from build123d import *

# Parameters (mm, degrees)
F0_W         = 35
F0_H         = 12
F0_W_2       = 12
F0_H_2       = 2
F1_DEPTH     = 0.6
F3_DEPTH     = 0.6
F4_R         = 2
F5_R         = 0.5
F6_SIZE      = 0.5
F7_T1_DEPTH  = 8
F7_T3_DEPTH  = 31
F7_T6_ANGLE  = 90
F7_T8_ANGLE  = 90
F7_T10_ANGLE = 90
F7_T12_ANGLE = 90
F8_R         = 0.2


# Not quite as in the source:
# - a fillet or chamfer that OpenCascade refuses, or shapes differently, is made with other operations: its cross-section is extruded or revolved along the edge and cut away or added


with BuildPart() as f1:
    # F0 (on Top) → F1 (new body)
    with BuildSketch(Plane.XY):
        Rectangle(F0_W, F0_H)
        Rectangle(F0_W_2, F0_H_2, mode=Mode.SUBTRACT)
    extrude(amount=F1_DEPTH)

    # F2 (on face) → F3 (join)
    with BuildSketch(Plane.XY.offset(0.6)):
        Polygon((-6.8, 0), (-6, 0), (-6, 1), (6, 1), (6, 0), (6.8, 0), (6.8, 1.8), (-6.8, 1.8), align=None)
    extrude(amount=F3_DEPTH)

    # F4
    f4_edges = [f1.edges().sort_by_distance(p)[0] for p in [
        (-17.5, -6, 0.3),
        (-17.5, 6, 0.3),
        (17.5, 6, 0.3),
        (17.5, -6, 0.3),
    ]]
    fillet(f4_edges, radius=F4_R)

    # F5
    f5_edges = [f1.edges().sort_by_distance(p)[0] for p in [
        (6.8, 1.8, 0.9),
        (6.8, 0, 0.9),
        (-6.8, 1.8, 0.9),
        (-6.8, 0, 0.9),
    ]]
    fillet(f5_edges, radius=F5_R)

    # F6
    f6_edges = [f1.edges().sort_by_distance(p)[0] for p in [
        (0, -1, 0.6),
    ]]
    chamfer(f6_edges, length=F6_SIZE)

    # F7: fillet of radius 0.8 on 8 edges, made by hand

    # F7_s2 → F7_t1 (cut)
    with BuildSketch(Plane.XZ.offset(-4)):
        with BuildLine():
            ThreePointArc((16.7254033308, 0.6), (17.2153012793, 0.432455532), (17.5, 0))
            Line((17.5, 0), (17.5, 0.6))
            Line((17.5, 0.6), (16.7254033308, 0.6))
        make_face()
        with BuildLine():
            ThreePointArc((-16.7254033308, 0.6), (-17.2153012793, 0.432455532), (-17.5, 0))
            Line((-17.5, 0), (-17.5, 0.6))
            Line((-17.5, 0.6), (-16.7254033308, 0.6))
        make_face()
    extrude(amount=F7_T1_DEPTH, mode=Mode.SUBTRACT)

    # F7_s4 → F7_t3 (cut)
    with BuildSketch(Plane.YZ.offset(-15.5)):
        with BuildLine():
            ThreePointArc((5.2254033308, 0.6), (5.7153012793, 0.432455532), (6, 0))
            Line((6, 0), (6, 0.6))
            Line((6, 0.6), (5.2254033308, 0.6))
        make_face()
        with BuildLine():
            ThreePointArc((-5.2254033308, 0.6), (-5.7153012793, 0.432455532), (-6, 0))
            Line((-6, 0), (-6, 0.6))
            Line((-6, 0.6), (-5.2254033308, 0.6))
        make_face()
    extrude(amount=F7_T3_DEPTH, mode=Mode.SUBTRACT)

    # F7_s5 → F7_t6 (revolve, cut)
    with BuildSketch(Plane.YZ.offset(15.5)):
        with BuildLine():
            ThreePointArc((5.2254033308, 0.6), (5.7153012793, 0.432455532), (6, 0))
            Line((6, 0), (6, 0.6))
            Line((6, 0.6), (5.2254033308, 0.6))
        make_face()
    revolve(axis=Axis((15.5, 4, 0.6), (0, 0, -1)), revolution_arc=F7_T6_ANGLE, mode=Mode.SUBTRACT)

    # F7_s7 → F7_t8 (revolve, cut)
    with BuildSketch(Plane.YZ.offset(15.5)):
        with BuildLine():
            ThreePointArc((-5.2254033308, 0.6), (-5.7153012793, 0.432455532), (-6, 0))
            Line((-6, 0), (-6, 0.6))
            Line((-6, 0.6), (-5.2254033308, 0.6))
        make_face()
    revolve(axis=Axis((15.5, -4, 0.6), (0, 0, 1)), revolution_arc=F7_T8_ANGLE, mode=Mode.SUBTRACT)

    # F7_s9 → F7_t10 (revolve, cut)
    with BuildSketch(Plane.YZ.offset(-15.5)):
        with BuildLine():
            ThreePointArc((-5.2254033308, 0.6), (-5.7153012793, 0.432455532), (-6, 0))
            Line((-6, 0), (-6, 0.6))
            Line((-6, 0.6), (-5.2254033308, 0.6))
        make_face()
    revolve(axis=Axis((-15.5, -4, 0.6), (0, 0, -1)), revolution_arc=F7_T10_ANGLE, mode=Mode.SUBTRACT)

    # F7_s11 → F7_t12 (revolve, cut)
    with BuildSketch(Plane.YZ.offset(-15.5)):
        with BuildLine():
            ThreePointArc((5.2254033308, 0.6), (5.7153012793, 0.432455532), (6, 0))
            Line((6, 0), (6, 0.6))
            Line((6, 0.6), (5.2254033308, 0.6))
        make_face()
    revolve(axis=Axis((-15.5, 4, 0.6), (0, 0, 1)), revolution_arc=F7_T12_ANGLE, mode=Mode.SUBTRACT)

    # F8
    f8_edges = [f1.edges().sort_by_distance(p)[0] for p in [
        (6.15, 0, 1.2),
        (6.653553, 0.146447, 1.2),
        (6.8, 0.9, 1.2),
        (6.653553, 1.653553, 1.2),
        (0, 1.8, 1.2),
        (-6.653553, 1.653553, 1.2),
        (-6.8, 0.9, 1.2),
        (-6.653553, 0.146447, 1.2),
        (-6.15, 0, 1.2),
        (-6, 0.5, 1.2),
        (0, 1, 1.2),
        (6, 0.5, 1.2),
    ]]
    fillet(f8_edges, radius=F8_R)


solid = f1.part
Read the model definition and answer for the solid it produces. Units are mm, in the model's axes. A direction names the side the tool comes from. Give positions to 0.01 mm unless a question says otherwise; leave off trailing zeros. Loops run counter-clockwise (first coordinate to the right, second up) from the corner with the lowest first, then second, coordinate; pieces in that order, holes last. Notation, with made-up numbers: M 83,26.5 L 131,26.5 A23 ccw 131,49.5 Z; hole C 0,11 d9. An arc over 180 degrees is marked long. Write each question's results on one line, items separated by ' | '.
1. Section D-D on x = 10.5 is taken. Give the vertices of the cut face in (y, z).
Values:
outline: M -6,0 L 6,0 A0.8 ccw 5.23,0.6 L -5.23,0.6 A0.8 ccw Z
2. A tool of negligible diameter and unlimited length cuts with its end or side. For faces 3 (the face through (0, 1.4, 1.2)), 4 (the face through (-0.1, 1, 0.5)), from which of +Z, -Z, +X, -X, +Y, -Y can it reach the whole face along a straight path? Write none if from no direction.
Values:
face 3: +Z, +X, -X, +Y, -Y | face 4: +Z, -Z
3. The mould has two halves that part along X. Classify faces 1 (the face through (6, 0, 0.4)), 2 (the face through (0, 2, 0.6)): pulls with the +X half, pulls with the -X half, needs draft (parallel to the pull), parting line crosses it, or undercut.
Values:
face 1: undercut | face 2: needs draft
4. Section A-A on x = 3 is taken. Give the vertices of the cut face in (y, z).
Values:
outline: M -6,0 L -1,0 L -1,0.1 L -1.5,0.6 L -5.23,0.6 A0.8 ccw Z; M 1,0 L 6,0 A0.8 ccw 5.23,0.6 L 1.8,0.6 L 1.8,1 A0.2 ccw 1.6,1.2 L 1.2,1.2 A0.2 ccw 1,1 Z
5. Given pin 1 (0.5 mm diameter, centred on y = 0, z = 0.5, fed in from +X); pin 2 (6 mm diameter, centred on x = 4, y = -3, fed in from +Z); pin 3 (5 mm diameter, centred on x = 5.5, y = 0, fed in from +Z), each flat-ended and moving along its own axis, determine where each tip first touches the part or whether it passes through.
Values:
pin 1: stops at x = 17.39 | pin 2: stops at z = 0.6 | pin 3: stops at z = 1.2
6. Straight lines are drawn through the part: line 1 (X direction, y = 0.75, z = 0.9); line 2 (Z direction, x = 9, y = 2); line 3 (X direction, y = 0.25, z = 1.15). For each, find the intervals that lie inside material, in ascending order. Write a range as [from, to].
Values:
line 1: x = [-6.8, -6], [6, 6.8] | line 2: z = [0, 0.6] | line 3: x = [-6.65, -6.07], [6.07, 6.65]
7. Section B-B on z = 0.3 is taken. Give the vertices of the cut face in (x, y), plus the area to 3 significant figures.
Values:
outline: M -17.35,-4 A1.85 ccw -15.5,-5.85 L 15.5,-5.85 A1.85 ccw 17.35,-4 L 17.35,4 A1.85 ccw 15.5,5.85 L -15.5,5.85 A1.85 ccw -17.35,4 Z; hole M -6,-1.2 L 6,-1.2 L 6,1 L -6,1 Z | area: 377 mm^2
8. Section C-C on y = -3.25 is taken. Give the vertices of the cut face in (x, z), plus the area to 3 significant figures.
Values:
outline: M -17.5,0 L 17.5,0 A0.8 ccw 16.73,0.6 L -16.73,0.6 A0.8 ccw Z | area: 20.8 mm^2
